Design review of the part built by this model. Coordinates are the model's own, in mm. A direction names the side the tool comes from. Coordinates: 2 decimals unless noted, no trailing zeros. Loops run counter-clockwise (first coordinate to the right, second up) from the corner with the lowest first, then second, coordinate; pieces in that order, holes last.
Q1. Wall thickness on probe 1 along X at (y, z) = (50, 48); probe 2 along X at (y, z) = (50, 79); probe 3 along Y at (x, z) = (49, 74.5): over which ranges is each line inside the solid? List them lowest first.
Q2. Draft analysis for pull direction X (two halves, no side actions). For faces 1 (the face through (61, 50, 20)), 2 (the face through (122.34, 31.525, 74.79)), 3 (the face through (21, 80, 65)), 4 (the face through (47.83, 40.24, 10.14)), state which applies: released by +X, released by -X, zero draft, split by the parting line, or undercut.
Q3. Machinability: for faces 5 (the face through (89, 90, 80)), 6 (the face through (170, 50, 73)), 7 (the face through (127.83, 40.24, 64.65)), 8 (the face through (100, 55, 73)), which of the approach directions +Z, -Z, +X, -X, +Y, -Y give a long, thin tool a straight path to every point of the face, cutting with its end or side? Answer none if there is none.
Q4. Add section A-A on z = 73. Give the boundary of the cut face in (x, y).
Q5. Add section B-B on z = 55. Give the boundary of the cut face in (x, y), and give its area (3 significant figures).
Q6. Add section D-D on y = 68. Give the boundary of the cut face in (x, z), and give its area (3 significant figures).
Q7. Add section C-C on x = 47. Give the boundary of the cut face in (y, z).
Q8. For P1, Ø10, axis at x = 149.5, z = 50, coming from the +Y side; P2, Ø12, axis at y = 36.5, z = 55.5, coming from the +X side; P3, Ø6, axis at x = 161.5, z = 73, coming from the +Y side, all flat-tipped, find the tip position at first contact; note any pin that passes through.
```python
from build123d import *

# Parameters (mm, degrees)
BOSS_EXTRUDE1_DEPTH        = 80
SKETCH2_W                  = 20
SKETCH2_H                  = 10
CUT_EXTRUDE1_DEPTH         = 209
SKETCH3_R                  = 10
CUT_EXTRUDE2_DEPTH         = 40
SKETCH4_R                  = 20
SKETCH4_R_2                = 10
BOSS_EXTRUDE2_DEPTH        = 10
F_20_0MM_DOWEL_HOLE1_D     = 20
F_20_0MM_DOWEL_HOLE1_DEPTH = 50
F_20_0MM_DOWEL_HOLE1_TIP   = 6.00860619
CUT_EXTRUDE3_DEPTH         = 20
SKETCH10_R                 = 10
CUT_EXTRUDE4_DEPTH         = 74
SKETCH11_R                 = 25
SKETCH11_R_2               = 10
CUT_EXTRUDE5_DEPTH         = 40
SKETCH12_R                 = 25
CUT_EXTRUDE6_DEPTH         = 10
SKETCH14_R                 = 35
SKETCH14_R_2               = 25
CUT_EXTRUDE7_DEPTH         = 30
SKETCH15_R                 = 35
CUT_EXTRUDE8_DEPTH         = 30
CUT_EXTRUDE9_DEPTH         = 20
SKETCH17_W                 = 20
SKETCH17_H                 = 5
BOSS_EXTRUDE3_DEPTH        = 25
SKETCH18_W                 = 20
SKETCH18_H                 = 5
BOSS_EXTRUDE4_DEPTH        = 25
SKETCH19_W                 = 20
SKETCH19_H                 = 5
BOSS_EXTRUDE5_DEPTH        = 25


with BuildPart() as part:
    # Sketch1 → Boss-Extrude1 (new body)
    with BuildSketch(Plane.XY):
        with BuildLine():
            ThreePointArc((0, 50), (14.644660941, 14.644660941), (50, 0))
            Line((50, 0), (130, 0))
            ThreePointArc((130, 0), (165.355339059, 14.644660941), (180, 50))
            ThreePointArc((180, 50), (165.355339059, 85.355339059), (130, 100))
            Line((130, 100), (50, 100))
            ThreePointArc((50, 100), (14.644660941, 85.355339059), (0, 50))
        make_face()
    extrude(amount=BOSS_EXTRUDE1_DEPTH)

    # Sketch2 → Cut-Extrude1 (cut)
    with BuildSketch(Plane(origin=(0, 0, 0), x_dir=(0, 0, -1), z_dir=(1, 0, 0))):
        with Locations((-70, 75)):
            Rectangle(SKETCH2_W, SKETCH2_H)
        with Locations((-70, 25)):
            Rectangle(SKETCH2_W, SKETCH2_H)
    extrude(amount=CUT_EXTRUDE1_DEPTH, mode=Mode.SUBTRACT)

    # Sketch3 → Cut-Extrude2 (cut)
    with BuildSketch(Plane.XY.offset(80)):
        with Locations((130, 50)):
            Circle(SKETCH3_R)
    extrude(amount=-CUT_EXTRUDE2_DEPTH, mode=Mode.SUBTRACT)

    # Sketch4 → Boss-Extrude2 (add)
    with BuildSketch(Plane.XY.offset(80)):
        with Locations(Location((130, 50, 0), (0, 0, 270))):
            Circle(SKETCH4_R)
        with Locations((130, 50)):
            Circle(SKETCH4_R_2, mode=Mode.SUBTRACT)
    extrude(amount=BOSS_EXTRUDE2_DEPTH)

    # Ø20.0mm Dowel Hole1
    with Locations(Plane(origin=(130, 50, 90), x_dir=(1, 0, 0), z_dir=(0, 0, 1))):
        with Locations((0, 0)):
            Hole(F_20_0MM_DOWEL_HOLE1_D / 2, depth=F_20_0MM_DOWEL_HOLE1_DEPTH)
            with Locations((0, 0, -(F_20_0MM_DOWEL_HOLE1_DEPTH + F_20_0MM_DOWEL_HOLE1_TIP / 2))):  # 118° drill point
                Cone(0, F_20_0MM_DOWEL_HOLE1_D / 2, F_20_0MM_DOWEL_HOLE1_TIP, mode=Mode.SUBTRACT)

    # Sketch9 → Cut-Extrude3 (cut)
    with BuildSketch(Plane.XY.offset(80)):
        with BuildLine():
            Line((130, 70), (4.17424305, 70))
            ThreePointArc((4.17424305, 70), (0, 50), (4.17424305, 30))
            Line((4.17424305, 30), (130, 30))
            ThreePointArc((130, 30), (110, 50), (130, 70))
        make_face()
    extrude(amount=-CUT_EXTRUDE3_DEPTH, mode=Mode.SUBTRACT)

    # Sketch10 → Cut-Extrude4 (cut)
    with BuildSketch(Plane.XY.offset(60)):
        with Locations((50, 50)):
            Circle(SKETCH10_R)
    extrude(amount=-CUT_EXTRUDE4_DEPTH, mode=Mode.SUBTRACT)

    # Sketch11 → Cut-Extrude5 (cut)
    with BuildSketch(Plane.XY.offset(60)):
        with Locations((50, 50)):
            Circle(SKETCH11_R)
        with Locations((50, 50)):
            Circle(SKETCH11_R_2, mode=Mode.SUBTRACT)
    extrude(amount=-CUT_EXTRUDE5_DEPTH, mode=Mode.SUBTRACT)

    # Sketch12 → Cut-Extrude6 (cut)
    with BuildSketch(Plane.XY.offset(60)):
        with BuildLine():
            Line((70, 80), (10, 80))
            ThreePointArc((10, 80), (0, 50), (10, 20))
            Line((10, 20), (70, 20))
            ThreePointArc((70, 20), (86.055512755, 50), (70, 80))
        make_face()
        with Locations((50, 50)):
            Circle(SKETCH12_R, mode=Mode.SUBTRACT)
    extrude(amount=-CUT_EXTRUDE6_DEPTH, mode=Mode.SUBTRACT)

    # Sketch14 → Cut-Extrude7 (cut)
    with BuildSketch(Plane.XY.offset(60)):
        with Locations((50, 50)):
            Circle(SKETCH14_R)
        with Locations((50, 50)):
            Circle(SKETCH14_R_2, mode=Mode.SUBTRACT)
    extrude(amount=-CUT_EXTRUDE7_DEPTH, mode=Mode.SUBTRACT)

    # Sketch15 → Cut-Extrude8 (cut)
    with BuildSketch(Plane.XY.offset(80)):
        with Locations((50, 50)):
            Circle(SKETCH15_R)
    extrude(amount=-CUT_EXTRUDE8_DEPTH, mode=Mode.SUBTRACT)

    # Sketch16 → Cut-Extrude9 (cut)
    with BuildSketch(Plane.XY.offset(80)):
        with BuildLine():
            Line((130, 70), (175.82575695, 70))
            ThreePointArc((175.82575695, 70), (180, 50), (175.82575695, 30))
            Line((175.82575695, 30), (130, 30))
            ThreePointArc((130, 30), (150, 50), (130, 70))
        make_face()
    extrude(amount=-CUT_EXTRUDE9_DEPTH, mode=Mode.SUBTRACT)

    # Sketch17 → Boss-Extrude3 (add)
    with BuildSketch(Plane.XY.offset(60)):
        with BuildLine():
            Line((150, 45), (150, 50))
            ThreePointArc((150, 50), (149.840593925, 47.47991415), (149.364916731, 45))
            Line((149.364916731, 45), (150, 45))
        make_face()
        with Locations((160, 47.5)):
            Rectangle(SKETCH17_W, SKETCH17_H)
        with BuildLine():
            ThreePointArc((110.635083269, 45), (110.159406075, 47.47991415), (110, 50))
            Line((110, 50), (110, 45))
            Line((110, 45), (110.635083269, 45))
        make_face()
        with Locations((100, 47.5)):
            Rectangle(SKETCH17_W, SKETCH17_H)
    extrude(amount=BOSS_EXTRUDE3_DEPTH)

    # Sketch18 → Boss-Extrude4 (add)
    with BuildSketch(Plane.XY.offset(85)):
        with BuildLine():
            ThreePointArc((110.635083269, 55), (110.159406075, 52.52008585), (110, 50))
            Line((110, 50), (110, 55))
            Line((110, 55), (110.635083269, 55))
        make_face()
        with Locations((100, 52.5)):
            Rectangle(SKETCH18_W, SKETCH18_H)
    extrude(amount=-BOSS_EXTRUDE4_DEPTH)

    # Sketch19 → Boss-Extrude5 (add)
    with BuildSketch(Plane.XY.offset(85)):
        with BuildLine():
            Line((150, 55), (149.364916731, 55))
            ThreePointArc((149.364916731, 55), (149.840593925, 52.52008585), (150, 50))
            Line((150, 50), (150, 55))
        make_face()
        with Locations((160, 52.5)):
            Rectangle(SKETCH19_W, SKETCH19_H)
    extrude(amount=-BOSS_EXTRUDE5_DEPTH)


solid = part.part
```
Entries:
1. probe 1: x = 0 to 15, 85 to 120, 140 to 180
1. probe 2: x = 90 to 120, 140 to 170
1. probe 3: y = 0.01 to 15.01, 84.99 to 99.99
2. face 1: undercut
2. face 2: split by the parting line
2. face 3: zero draft
2. face 4: undercut
3. face 5: +Z, +X, -X, +Y
3. face 6: +Z, +X, +Y, -Y
3. face 7: +Z
3. face 8: +Z, -X
4. outline: (10, 20) arc R50 ccw to (50, 0) - (130, 0) arc R50 ccw to (170, 20) - (68.03, 20) arc R35 cw to (31.97, 20) - close; (10, 80) - (31.97, 80) arc R35 cw to (68.03, 80) - (170, 80) arc R50 ccw to (130, 100) - (50, 100) arc R50 ccw to start; (90, 45) - (110.64, 45) arc R20 ccw to (149.36, 45) - (170, 45) - (170, 55) - (149.36, 55) arc R20 ccw to (110.64, 55) - (90, 55) - close; hole circle Ø20 at (130, 50)
5. outline: (10, 20) arc R50 ccw to (50, 0) - (130, 0) arc R50 ccw to (130, 100) - (50, 100) arc R50 ccw to (10, 80) - (31.97, 80) arc R35 cw to (68.03, 80) - (70, 80) arc R36.06 cw to (70, 20) - (68.03, 20) arc R35 cw to (31.97, 20) - close; hole circle Ø20 at (130, 50)
5. area: 10,600 mm2
6. outline: (3.35, 0) - (176.65, 0) - (176.65, 60) - (138.72, 60) - (138.72, 90) - (121.28, 90) - (121.28, 60) - (81.24, 60) - (81.24, 50) - (80.02, 50) - (80.02, 30) - (67.35, 30) - (67.35, 20) - (32.65, 20) - (32.65, 30) - (19.98, 30) - (19.98, 50) - (3.35, 50) - close
6. area: 8,590 mm2
7. outline: (0.09, 0) - (40.46, 0) - (40.46, 20) - (25.18, 20) - (25.18, 30) - (15.13, 30) - (15.13, 80) - (0.09, 80) - close; (59.54, 0) - (99.91, 0) - (99.91, 80) - (84.87, 80) - (84.87, 30) - (74.82, 30) - (74.82, 20) - (59.54, 20) - close
8. P1: stops at y = 97.85
8. P2: stops at x = 179.43
8. P3: stops at y = 91.08
